from build123d import *

# Parameters (mm, degrees)
F0_W     = 140
F0_H     = 25.4
F1_DEPTH = 61.9
F3_DEPTH = 12.7
F4_R     = 2
F5_DEPTH = 3.5


with BuildPart() as f1:
    # F0 (on Front) → F1 (new body)
    with BuildSketch(Plane.XZ):
        with Locations((10.794906, -20.302821)):
            Rectangle(F0_W, F0_H)
    extrude(amount=F1_DEPTH)

    # F2 (on face) → F3 (cut)
    with BuildSketch(Plane(origin=(0, 0, -33.002821), x_dir=(1, 0, 0), z_dir=(0, 0, -1))):
        Polygon((-55.205094, 0), (44.794906, 0), (44.794906, 60), (80.794906, 60), (80.794906, 61.9), (-59.205094, 61.9), (-59.205094, 60), (-55.205094, 60), align=None)
    extrude(amount=-F3_DEPTH, mode=Mode.SUBTRACT)

    # F4 (on face) → F5 (join)
    with BuildSketch(Plane(origin=(0, 0, -20.302821), x_dir=(1, 0, 0), z_dir=(0, 0, -1))):
        with Locations((-27.430094, 48.824)):
            Circle(F4_R)
        with Locations((-27.430094, 36.124)):
            Circle(F4_R)
        with Locations((17.019906, 48.824)):
            Circle(F4_R)
        with Locations((17.019906, 36.124)):
            Circle(F4_R)
    extrude(amount=F5_DEPTH)


solid = f1.part
The model under review builds one solid part; all positions refer to its coordinate system, in mm. A direction names the side the tool comes from. Give positions to 0.01 mm unless a question says otherwise; leave off trailing zeros. Write each loop counter-clockwise with the first axis right and the second up, starting at its lowest first coordinate (ties: lowest second). Pieces come first, ordered by that corner, then holes.
1. Tool access review of faces 4 (the flat face through (17, -36, -23.803)), 5 (the flat face through (-57, -60, -27)), 6 (the cylindrical face through (-29.43, -36.21, -22.03)): name each direction out of +Z, -Z, +X, -X, +Y, -Y from which nothing blocks a thin tool from reaching the whole face with its end or side.
2. Add section A-A, the plane z = -25.25. Write out the cut boundary in (x, y), plus the area to 3 significant figures.
3. Wall thickness on L1, parallel to X at y = -39, z = -24.5; L2, parallel to Z at x = 34, y = -55; L3, parallel to Y at x = 75, z = -31: over which ranges is each line inside the solid? List them lowest first.
4. Add section C-C, the plane x = 68.5. Write out the cut boundary in (y, z), plus the area to 3 significant figures.
5. Add section B-B, the plane y = -17.5. Write out the cut boundary in (x, z), plus the area to 3 significant figures.
6. Draft analysis for pull direction X (two halves, no side actions). For faces 1 (the flat face through (63, -30, -33.003)), 2 (the flat face through (-27, -49, -23.803)), 3 (the flat face through (80.795, -31, -20)), state which applies: +X half, -X half, draft (parallel to the pull), parting line (faces both ways), or undercut.
7. Add section D-D, the plane x = 12. Write out the cut boundary in (y, z), plus the area to 3 significant figures.
8. For P1, Ø2, axis at x = 18, y = -49, coming from the -Z side; P2, Ø10, axis at x = 59, z = -29, coming from the -Y side; P3, Ø1, axis at x = 4, y = -34, coming from the -Z side, all flat-tipped, find the tip position at first contact; note any pin that passes through.
Worked answers:
1. face 4: -Z, +Y, -Y
1. face 5: -Z, +X, -X, -Y
1. face 6: -Z
2. outline: (-59.21, -60) - (-55.21, -60) - (-55.21, 0) - (-59.21, 0) - close; (44.79, -60) - (80.79, -60) - (80.79, 0) - (44.79, 0) - close
2. area: 2,400 mm2
3. L1: x = -59.21 to -55.21, 44.79 to 80.79
3. L2: z = -20.3 to -7.6
3. L3: y = -60 to 0
4. outline: (-61.9, -20.3) - (-60, -20.3) - (-60, -33) - (0, -33) - (0, -7.6) - (-61.9, -7.6) - close
4. area: 1,550 mm2
5. outline: (-59.21, -33) - (-55.21, -33) - (-55.21, -20.3) - (44.79, -20.3) - (44.79, -33) - (80.79, -33) - (80.79, -7.6) - (-59.21, -7.6) - close
5. area: 2,290 mm2
6. face 1: draft
6. face 2: undercut
6. face 3: +X half
7. outline: (-61.9, -20.3) - (0, -20.3) - (0, -7.6) - (-61.9, -7.6) - close
7. area: 786 mm2
8. P1: stops at z = -23.8
8. P2: stops at y = -60
8. P3: stops at z = -20.3
